Autodesk Inventor part; units mm, degrees
ref_plane "YZ Plane" through (0, 0, 0) normal (1, 0, 0) x (0, 1, 0)
ref_plane "XZ Plane" through (0, 0, 0) normal (0, 1, 0) x (-1, 0, 0)
ref_plane "XY Plane" through (0, 0, 0) normal (0, 0, 1) x (1, 0, 0)
sketch "hole pattern" plane through (0, 0, 0) normal (0, 0, 1) x (1, 0, 0)
  circle A0 centre (-54.635, 0) radius 5 construction
  line L0 (-126, 0) -> (126, 0)
  line L1 (0, -46) -> (0, 52)
  circle A1 centre (0, 5.5) radius 22.5
  line L2 (-54.635, -5) -> (0, -5) construction
  circle A2 centre (54.635, 0) radius 5 construction
  line L3 (-90, 38) -> (90, 38)
  line L4 (-90, 38) -> (-75, -32)
  line L5 (-75, -32) -> (75, -32)
  line L6 (75, -32) -> (90, 38)
  circle A3 centre (-54.635, 0) radius 15 construction
  circle A4 centre (54.635, 0) radius 15 construction
  circle A5 centre (-54.635, 0) radius 5.5
  circle A6 centre (54.635, 0) radius 5.5
  point P0 (0, 0)
  dimension "d1" = 10
  dimension "d0" = 54.635
  dimension "d2" = 45
  dimension "topWidth" = 180
  dimension "d38" = 90
  dimension "d39" = 32.5
  dimension "d40" = 10.5
  dimension "d41" = 32
  dimension "d42" = 30
  dimension "d43" = 30
  dimension "d44" = 11
  dimension "d45" = 11
  dimension "d76" = 150
extrude "Extrusion1" add sketch "hole pattern" along normal blind 15 contours L4 L3 L1 A1 L0 A5 | L0 A5 A1 L1 L5 L4 | L3 L6 L0 A6 A1 L1 | L1 A1 L0 A6 L6 L5
fillet "Fillet1" radius 2 2 edges at (-90, 38, 7.5) (90, 38, 7.5)
equation "\"d38\" = 0.5 * topWidth"
properties part number "Brake_Light_Base_Plate"
Geometry check sheet. Reference: the model listing, model coordinates, mm. Round coordinates to 2 decimals unless told otherwise and drop trailing zeros. Order: outer loops, then holes, each group sorted by start corner. A loop starts at its lowest first (then second) coordinate and runs counter-clockwise, first axis right, second up. Notation, with made-up numbers: M 46.5,58 L 85.5,58 A21 cw 85.5,93 Z; hole C 39,85.25 d7. An arc over 180 degrees is marked long. Write each question's results on one line, items separated by ' | '. Start each with the question number.
1. Cross-section at A-A on x = 0. Record the boundary of the cut face in (y, z), plus the area to 3 significant figures.
2. Cross-section at B-B on z = 11.75. Record the boundary of the cut face in (x, y) (3 decimals), plus the area to 3 significant figures.
3. Cross-section at D-D on y = 0. Record the boundary of the cut face in (x, z) (3 decimals), plus the area to 3 significant figures.
4. Draft check along X on faces 1 (the face through (-60.13, -0.24, 7.4)), 2 (the face through (-1, 38, 7)), 3 (the face through (82.14, 1.32, 7.4)). Enter one of: pulls with the +X half, pulls with the -X half, needs draft (parallel to the pull), parting line crosses it, or undercut.
5. Material ranges on L1, parallel to Y at x = 0, z = 7; L2, parallel to X at y = 0, z = 6.25 (3 decimals); L3, parallel to Y at x = -8.5, z = 8, recorded low to high. Write a range as from..to.
6. Cross-section at C-C on y = 9. Record the boundary of the cut face in (x, z), plus the area to 3 significant figures.
7. Go/stop test with flat-tipped pins: P1, Ø1.5, axis at y = -10.5, z = 3, coming from the -X side; P2, Ø5, axis at y = -9.5, z = 11.5, coming from the -X side. Record where each tip stops, or that it passes through.
Resolved:
1) outline: M -32,0 L -17,0 L -17,15 L -32,15 Z; M 28,0 L 38,0 L 38,15 L 28,15 Z | area: 375 mm2
2) outline: M -89.482,35.581 L -75,-32 L 75,-32 L 89.482,35.581 A2 ccw 87.526,38 L -87.526,38 A2 ccw Z; hole C -54.635,0 d11; hole C 0,5.5 d45; hole C 54.635,0 d11 | area: 9,770 mm2
3) outline: M -81.857,0 L -60.135,0 L -60.135,15 L -81.857,15 Z; M -49.135,0 L -21.817,0 L -21.817,15 L -49.135,15 Z; M 21.817,0 L 49.135,0 L 49.135,15 L 21.817,15 Z; M 60.135,0 L 81.857,0 L 81.857,15 L 60.135,15 Z | area: 1,470 mm2
4) face 1: undercut | face 2: needs draft | face 3: pulls with the +X half
5) L1: -32..-17, 28..38 | L2: -81.857..-60.135, -49.135..-21.817, 21.817..49.135, 60.135..81.857 | L3: -32..-15.33, 26.33..38
6) outline: M -83.79,0 L -22.23,0 L -22.23,15 L -83.79,15 Z; M 22.23,0 L 83.79,0 L 83.79,15 L 22.23,15 Z | area: 1,850 mm2
7) P1: x = -79.77 | P2: x = -80.36
